Source: CAD feature listing. Evaluate the final solid. Frame: model axes, mm. A direction names the side the tool comes from. Coordinates: 2 decimals unless noted, no trailing zeros. Order: outer loops, then holes, each group sorted by start corner. A loop starts at its lowest first (then second) coordinate and runs counter-clockwise, first axis right, second up.
Item 1: Contact query for flat-ended pins moving along their axis: P1, Ø8, axis at y = -88.5, z = 0.5, coming from the +X side; P2, Ø5.5, axis at x = 6, z = -5.5, coming from the +Y side; P3, Ø2, axis at x = 18.5, y = -74.5, coming from the +Z side. Output: stop coordinate, or through.
Item 2: Ray query, line 1 (X direction, y = -113, z = -0.75); line 2 (Z direction, x = 0, y = -96.5); line 3 (Z direction, x = 173, y = -31). Return the intervals inside material, ascending.
Item 3: Section A-A on x = 0. Return the cut outline in (y, z).
Item 4: Reachability of faces 5 (the flat face through (0, 0, -6)), 6 (the flat face through (-20, -76, 0)), 7 (the flat face through (0, 0, 6)) from +Z, -Z, +X, -X, +Y, -Y: full face, straight path, thin tool, end or side. Return the list, or none.
Item 5: Section C-C on x = 59.5. Return the cut outline in (y, z), then the cut area to 3 significant figures.
Item 6: Mould query, pull axis Z, two halves, no side actions, for faces 1 (the flat face through (-5, -158, 3)), 2 (the cylindrical face through (0.171, -77.894, 7.524)), 3 (the cylindrical face through (5.244, -77.894, -2.174)), 4 (the cylindrical face through (-0.171, -77.894, -7.524)). Classes: released by +Z, released by -Z, zero draft, split by the parting line, or undercut.
Item 7: Section B-B on y = -83. Return the cut outline in (x, z).
from build123d import *

# Parameters (mm, degrees)
F0_R     = 5.676649
F1_DEPTH = 158
F2_W     = 3
F2_H     = 1
F2_W_2   = 37
F3_DEPTH = 300
F4_W     = 0.3
F4_H     = 9
F5_DEPTH = 0.5


with BuildPart() as f1:
    # F0 (on Front) → F1 (new body)
    with BuildSketch(Plane.XZ):
        with BuildLine():
            Line((17.630959, -5.5), (19.5, -5.5))
            ThreePointArc((19.5, -5.5), (19.853553, -5.353553), (20, -5))
            Line((20, -5), (20, 5))
            ThreePointArc((20, 5), (19.853553, 5.353553), (19.5, 5.5))
            Line((19.5, 5.5), (17.630959, 5.5))
            ThreePointArc((17.630959, 5.5), (17.007706, 5.451146), (16.399678, 5.305778))
            Line((16.399678, 5.305778), (14.734471, 4.767035))
            ThreePointArc((14.734471, 4.767035), (13.268353, 4.579712), (11.834298, 4.937596))
            ThreePointArc((11.834298, 4.937596), (0, 7.524315), (-11.834298, 4.937596))
            ThreePointArc((-11.834298, 4.937596), (-13.268353, 4.579712), (-14.734471, 4.767035))
            Line((-14.734471, 4.767035), (-16.399678, 5.305778))
            ThreePointArc((-16.399678, 5.305778), (-17.007706, 5.451146), (-17.630959, 5.5))
            Line((-17.630959, 5.5), (-19.5, 5.5))
            ThreePointArc((-19.5, 5.5), (-19.853553, 5.353553), (-20, 5))
            Line((-20, 5), (-20, -5))
            ThreePointArc((-20, -5), (-19.853553, -5.353553), (-19.5, -5.5))
            Line((-19.5, -5.5), (-17.630959, -5.5))
            ThreePointArc((-17.630959, -5.5), (-17.007706, -5.451146), (-16.399678, -5.305778))
            Line((-16.399678, -5.305778), (-14.734471, -4.767035))
            ThreePointArc((-14.734471, -4.767035), (-13.268353, -4.579712), (-11.834298, -4.937596))
            ThreePointArc((-11.834298, -4.937596), (0, -7.524315), (11.834298, -4.937596))
            ThreePointArc((11.834298, -4.937596), (13.268353, -4.579712), (14.734471, -4.767035))
            Line((14.734471, -4.767035), (16.399678, -5.305778))
            ThreePointArc((16.399678, -5.305778), (17.007706, -5.451146), (17.630959, -5.5))
        make_face()
        Circle(F0_R, mode=Mode.SUBTRACT)
    extrude(amount=F1_DEPTH)

    # F2 (on face) → F3 (join)
    with BuildSketch(Plane(origin=(-20, 0, 0), x_dir=(0, -1, 0), z_dir=(-1, 0, 0))):
        with Locations((-1.5, 0)):
            Rectangle(F2_W, F2_H)
        with Locations((18.5, 0)):
            Rectangle(F2_W_2, F2_H)
    extrude(amount=-F3_DEPTH)

    # F4 (on face) → F5 (cut)
    with BuildSketch(Plane.XY.offset(0.5)):
        with Locations((275.1, -1.5)):
            Rectangle(F4_W, F4_H)
    extrude(amount=-F5_DEPTH, mode=Mode.SUBTRACT)


solid = f1.part
Answer list:
1. P1: stops at x = 20
1. P2: stops at y = 0
1. P3: stops at z = 5.5
2. line 1: x = -20 to -5.63, 5.63 to 20
2. line 2: z = -7.52 to -5.68, 5.68 to 7.52
2. line 3: z = -0.5 to 0.5
3. outline: (-158, -7.52) - (0, -7.52) - (0, -5.68) - (-158, -5.68) - close; (-158, 5.68) - (0, 5.68) - (0, 7.52) - (-158, 7.52) - close; (-37, -0.5) - (3, -0.5) - (3, 0.5) - (-37, 0.5) - close
4. face 5: -Z, +X, -X, +Y
4. face 6: +Z, -Z, -X, +Y, -Y
4. face 7: +Z, +X, -X, +Y
5. outline: (-37, -0.5) - (3, -0.5) - (3, 0.5) - (-37, 0.5) - close
5. area: 40.0 mm2
6. face 1: zero draft
6. face 2: released by +Z
6. face 3: undercut
6. face 4: released by -Z
7. outline: (-20, -5) arc R0.5 ccw to (-19.5, -5.5) - (-17.63, -5.5) arc R4 ccw to (-16.4, -5.31) - (-14.73, -4.77) arc R4 cw to (-11.83, -4.94) arc R28.36 ccw to (11.83, -4.94) arc R4 cw to (14.73, -4.77) - (16.4, -5.31) arc R4 ccw to (17.63, -5.5) - (19.5, -5.5) arc R0.5 ccw to (20, -5) - (20, 5) arc R0.5 ccw to (19.5, 5.5) - (17.63, 5.5) arc R4 ccw to (16.4, 5.31) - (14.73, 4.77) arc R4 cw to (11.83, 4.94) arc R28.36 ccw to (-11.83, 4.94) arc R4 cw to (-14.73, 4.77) - (-16.4, 5.31) arc R4 ccw to (-17.63, 5.5) - (-19.5, 5.5) arc R0.5 ccw to (-20, 5) - close; hole circle Ø11.35 at (0, 0)
